Part model, mm, in its own coordinate system. A direction names the side the tool comes from. Round coordinates to 2 decimals unless told otherwise and drop trailing zeros. Loops run counter-clockwise (first coordinate to the right, second up) from the corner with the lowest first, then second, coordinate; pieces in that order, holes last. Notation, with made-up numbers: (73.5, 3.5) -> (89.5, 3.5) arc R20 ccw to (89.5, 8.5) -> close; hole circle Ø1 at (7.25, -34). An arc over 180 degrees is marked (long way). Answer as CSV lines item,"result".
from build123d import *

# Parameters (mm, degrees)
F1_DEPTH = 561.975
F2_R     = 2.6162
F4_DEPTH = 25.4
F3_R     = 2.6162
F5_DEPTH = 25.4


with BuildPart() as f1:
    # F0 (on Right) → F1 (new body)
    with BuildSketch(Plane.YZ):
        Polygon((0, -17.4625), (0, 0), (-1.5875, 0), (-1.5875, -19.05), (17.4625, -19.05), (17.4625, -17.4625), align=None)
    extrude(amount=-F1_DEPTH)

    # F2 (on face) → F4 (cut)
    with BuildSketch(Plane(origin=(0, 0, 0), x_dir=(-1, 0, 0), z_dir=(0, 1, 0))):
        with Locations((10.31875, -8.733851)):
            Circle(F2_R)
        with Locations((279.399963, -8.636074)):
            Circle(F2_R)
        with Locations((551.6626, -8.73125)):
            Circle(F2_R)
        with Locations((508, -8.553008)):
            Circle(F2_R)
        with Locations((50.8, -8.719141)):
            Circle(F2_R)
    extrude(amount=-F4_DEPTH, mode=Mode.SUBTRACT)

    # F3 (on face) → F5 (cut)
    with BuildSketch(Plane.XY.offset(-17.4625)):
        with Locations((-8.73125, 8.73125)):
            Circle(F3_R)
        with Locations((-553.24375, 8.73125)):
            Circle(F3_R)
    extrude(amount=-F5_DEPTH, mode=Mode.SUBTRACT)


solid = f1.part
Q1. Saw through at A-A, the plane x = -228. Write the cut outline in (y, z).
Geometry results:
outline,"(-1.59, -19.05) -> (17.46, -19.05) -> (17.46, -17.46) -> (0, -17.46) -> (0, 0) -> (-1.59, 0) -> close"
Q2. Drop flat-ended pins along their axis: P1, Ø8.5, axis at x = -10.32, z = -8.73, coming from the +Y side; P2, Ø8, axis at x = -433, y = 11.5, coming from the +Z side. Give the stop position or say it passes through.
Geometry results:
P1,"y = 0"
P2,"z = -17.46"
Q3. Which spindle directions (+Z, -Z, +X, -X, +Y, -Y) get a long thin tool onto all of the face, cutting with end or side? Do faces 1 (the face through (-277, 0, -7)), 2 (the face through (-277, -1.588, -12)). Say none if no direction does.
Geometry results:
face 1,"+Z, +X, -X, +Y"
face 2,"+Z, -Z, +X, -X, -Y"
Q4. Drill centre lines: line 1 along Z through (x, y) = (-508, -0.8); line 2 along Y through (x, z) = (-83, -8); line 3 along Z through (x, y) = (-313.5, 13.25). Where is each one in solid material? Low to high.
Geometry results:
line 1,"-19.05 to -11.17, -5.94 to 0"
line 2,"-1.59 to 0"
line 3,"-19.05 to -17.46"
